Part model, mm, in its own coordinate system. A direction names the side the tool comes from. Round coordinates to 2 decimals unless told otherwise and drop trailing zeros. Write each loop counter-clockwise with the first axis right and the second up, starting at its lowest first coordinate (ties: lowest second). Pieces come first, ordered by that corner, then holes. Notation, with made-up numbers: M -33,11.25 L -20,11.25 A13 ccw -20,25.25 Z; hole C 19.25,-35.5 d6. An arc over 180 degrees is marked long. Answer as a JSON object with one key per item and string values. Group by question number.
1. Two-plate mould, pull along X, no slides. Class faces 1 (the face through (57.839, -6.312, -3.131)), 2 (the face through (40, 122, -6.35)), 3 (the face through (43.75, 95.26, -3.13)): +X half, -X half, draft (parallel to the pull), parting line (faces both ways), or undercut.
2. Band-saw the part on C-C, the plane z = -4.5. Write the cut outline in (x, y), plus the area to 3 significant figures.
3. Drill centre lines: line 1 (X direction, y = 73.5, z = -1.75); line 2 (X direction, y = 143, z = -5.25); line 3 (Y direction, x = -11.5, z = -0.25). Where is each one in solid material? Low to high. Write a range as from..to.
4. Band-saw the part on B-B, the plane y = 113. Write the cut outline in (x, z), plus the area to 3 significant figures.
5. Band-saw the part on A-A, the plane x = 10. Write the cut outline in (y, z).
6. Drop flat-ended pins along their axis: pin 1 (1.5 mm diameter, centred on x = 21.5, z = -4.5, fed in from +Y); pin 2 (3 mm diameter, centred on y = 43.5, z = -2, fed in from +X); pin 3 (1 mm diameter, centred on x = 1.5, z = -1, fed in from +Y); pin 4 (6 mm diameter, centred on x = 42, y = 93.5, fed in from +Z). Give the stop position or say it passes through.
7. Which spindle directions (+Z, -Z, +X, -X, +Y, -Y) get a long thin tool onto all of the face, cutting with end or side? Do faces 4 (the face through (14.727, 84.199, -3.131)), 5 (the face through (10.72, 85.3, -3.13)). Say none if no direction does.
Autodesk Inventor part; units mm, degrees
ref_plane "YZ Plane" through (0, 0, 0) normal (1, 0, 0) x (0, 1, 0)
ref_plane "XZ Plane" through (0, 0, 0) normal (0, 1, 0) x (-1, 0, 0)
ref_plane "XY Plane" through (0, 0, 0) normal (0, 0, 1) x (1, 0, 0)
sketch "Sketch1" plane through (0, 0, 0) normal (0, 0, 1) x (1, 0, 0)
  line L0 (30.9216, 189.4198) -> (63.3973, -1.1372)
  line L1 (-28.8193, 170.8268) -> (51.3861, -2.6646)
  line L2 (27.7918, 188.8864) -> (60.1566, -1.0202)
  line L3 (54.2681, -1.3323) -> (-25.9374, 172.1591)
  arc A0 (54.2681, -1.3323) -> (60.1566, -1.0202) centre (57.15, 0) ccw
  arc A1 (51.3861, -2.6646) -> (63.3973, -1.1372) centre (57.15, 0) ccw
  arc A2 (27.7918, 188.8864) -> (-25.9374, 172.1591) centre (-0.1919, 184.1173) ccw
  arc A3 (30.9216, 189.4198) -> (-28.8193, 170.8268) centre (-0.1919, 184.1173) ccw
  point P0 (0, 0)
  point P1 (-0.3472, 183.9895)
  dimension "d4" = 3.175
extrude "Extrusion1" add sketch "Sketch1" against normal blind 6.35
properties part number "proxy chain 1"
Worked answers:
{
 "1": {"face 1": "parting line", "face 2": "draft", "face 3": "undercut"},
 "2": {"outline": "M -28.82,170.83 L 51.39,-2.66 A6.35 ccw 63.4,-1.14 L 30.92,189.42 A31.56 ccw long Z; hole M -25.94,172.16 L 54.27,-1.33 A3.17 ccw 60.16,-1.02 L 27.79,188.89 A28.39 ccw long Z", "area": "1,580 mm^2"},
 "3": {"line 1": "x = 16.18..19.67, 47.46..50.68", "line 2": "x = -15.95..-12.46, 35.61..38.83", "line 3": "y = 133.36..140.93, 210.15..213.58"},
 "4": {"outline": "M -2.09,-6.35 L 1.41,-6.35 L 1.41,0 L -2.09,0 Z; M 40.72,-6.35 L 43.95,-6.35 L 43.95,0 L 40.72,0 Z", "area": "42.7 mm^2"},
 "5": {"outline": "M 86.86,-6.35 L 94.42,-6.35 L 94.42,0 L 86.86,0 Z; M 210.61,-6.35 L 213.99,-6.35 L 213.99,0 L 210.61,0 Z"},
 "6": {"pin 1": "stops at y = 207.73", "pin 2": "stops at x = 56.05", "pin 3": "stops at y = 215.66", "pin 4": "stops at z = 0"},
 "7": {"face 4": "+Z, -Z", "face 5": "+Z, -Z, -X, -Y"}
}
